from build123d import *

# Parameters (mm, degrees)
F1_DEPTH  = 19.05
F4_DEPTH  = 114.3
F5_W      = 304.8
F5_H      = 76.2
F6_DEPTH  = 205.103861168
F8_DEPTH  = 762
F10_DEPTH = 762
F11_W     = 50.8
F11_H     = 50.8
F12_DEPTH = 762


with BuildPart() as f1:
    # F0 (on Top) → F1 (new body)
    with BuildSketch(Plane.XY):
        Polygon((609.6, 0), (0, 0), (0, -609.6), (76.1936366749, -610.5847488248), (609.6, -76.2), align=None)
    extrude(amount=F1_DEPTH)

    # F3 (on face) → F4 (join)
    with BuildSketch(Plane(origin=(0, 0, 0), x_dir=(1, 0, 0), z_dir=(0, 0, -1))):
        Polygon((584.2, 65.6926060926), (65.7952397089, 585.0482356184), (25.4, 584.5261557366), (25.4, 25.4), (584.2, 25.4), align=None)
        Polygon((44.45, 44.45), (44.45, 565.720772539), (57.9964419843, 565.8958507136), (565.15, 57.8120606621), (565.15, 44.45), align=None, mode=Mode.SUBTRACT)
    extrude(amount=F4_DEPTH)

    # F5 (on face) → F6 (cut)
    with BuildSketch(Plane(origin=(325.4815326726, -324.8856204339, 0), x_dir=(0.7064585835, 0.7077543852, 0), z_dir=(0.7077543852, -0.7064585835, 0))):
        with Locations((0, -57.15)):
            Rectangle(F5_W, F5_H)
    extrude(amount=-F6_DEPTH, mode=Mode.SUBTRACT)

    # F7 (on face) → F8 (join)
    with BuildSketch(Plane(origin=(0, 0, 0), x_dir=(1, 0, 0), z_dir=(0, 0, -1))):
        Polygon((57.9964419843, 565.8958507136), (44.45, 565.8958507136), (44.45, 515.0958507136), (107.8850816302, 515.9157042449), align=None)
    extrude(amount=F8_DEPTH)

    # F9 (on face) → F10 (join)
    with BuildSketch(Plane(origin=(0, 0, 0), x_dir=(1, 0, 0), z_dir=(0, 0, -1))):
        Polygon((565.15, 44.45), (565.15, 57.8120606621), (514.35, 108.7052391219), (514.35, 44.45), align=None)
    extrude(amount=F10_DEPTH)

    # F11 (on face) → F12 (join)
    with BuildSketch(Plane(origin=(0, 0, 0), x_dir=(1, 0, 0), z_dir=(0, 0, -1))):
        with Locations((69.85, 69.85)):
            Rectangle(F11_W, F11_H)
    extrude(amount=F12_DEPTH)


solid = f1.part
Geometry check sheet. Reference: the model listing, model coordinates, mm. A direction names the side the tool comes from. Coordinates: 2 decimals unless noted, no trailing zeros. Order: outer loops, then holes, each group sorted by start corner. A loop starts at its lowest first (then second) coordinate and runs counter-clockwise, first axis right, second up. Notation, with made-up numbers: (75.5, 15.25) - (131.5, 15.25) arc R22 cw to (131.5, 26.25) - close; hole circle Ø6 at (-37, 57.5). An arc over 180 degrees is marked (long way). Answer in a Markdown table with one row per item. Add a question column.
1) Cross-section at A-A, the plane z = -592. Record the cut outline in (x, y).
2) Release check for a two-part mould opening along Y. For faces 6 (the flat face through (534, -70, -762)), 7 (the flat face through (224, -224, 0)), 8 (the flat face through (83.29, -540.556, -433.616)) record: +Y half, -Y half, draft (parallel to the pull), parting line (faces both ways), or undercut.
3) Cross-section at B-B, the plane y = -325.5. Record the cut outline in (x, z), then the cut area to 3 significant figures.
4) Material ranges on line 1 along Z through (x, y) = (81, -341); line 2 along Z through (x, y) = (380.5, -255); line 3 along X through (y, z) = (-211.5, -28.5), recorded low to high. Write a range as [from, to].
5) Set-up check for faces 1 (the flat face through (301, -25.4, -56)), 2 (the flat face through (0, -301, 9)), 3 (the flat face through (540.11, -82.9, -433.62)), 4 (the flat face through (44.45, -69, -434)), 5 (the flat face through (584.2, -45, -56)): record each of +Z, -Z, +X, -X, +Y, -Y from which the full face is reachable in a straight line by a thin tool's end or side.
6) Cross-section at D-D, the plane z = -68. Record the cut outline in (x, y), then the cut area to 3 significant figures.
7) Cross-section at C-C, the plane x = 292.5. Record the cut outline in (y, z).
8) Gauge pin test, flat ends, axial feed: P1, Ø12, axis at x = 486, y = -93.5, coming from the -Z side; P2, Ø11, axis at x = 50, z = -498, coming from the -Y side; P3, Ø14.5, axis at y = -52.5, z = -506.5, coming from the +X side. Record the tip position at first contact, or that the pin passes through.
Check result:
| question | item | result |
|---|---|---|
| 1 | outline | (44.45, -565.9) - (58, -565.9) - (107.89, -515.92) - (44.45, -515.1) - close; (44.45, -95.25) - (95.25, -95.25) - (95.25, -44.45) - (44.45, -44.45) - close; (514.35, -108.71) - (565.15, -57.81) - (565.15, -44.45) - (514.35, -44.45) - close |
| 2 | face 6 | draft |
| 2 | face 7 | undercut |
| 2 | face 8 | -Y half |
| 3 | outline | (0, 0) - (25.4, 0) - (25.4, -114.3) - (44.45, -114.3) - (44.45, 0) - (297.95, 0) - (297.95, -19.05) - (324.87, -19.05) - (324.87, 0) - (360.76, 0) - (360.76, 19.05) - (0, 19.05) - close; (297.95, -114.3) - (324.87, -114.3) - (324.87, -95.25) - (297.95, -95.25) - close |
| 3 | area | 10,100 mm² |
| 4 | line 1 | z = [0, 19.05] |
| 4 | line 2 | z = [-114.3, -95.25], [-19.05, 19.05] |
| 4 | line 3 | x = [25.4, 44.45], [427.61, 438.66] |
| 5 | face 1 | -Z, +X, -X, +Y |
| 5 | face 2 | +Z, -Z, -X, +Y, -Y |
| 5 | face 3 | -Z, +X, -Y |
| 5 | face 4 | -Z, -X, +Y, -Y |
| 5 | face 5 | -Z, +X, +Y, -Y |
| 6 | outline | (25.4, -584.53) - (65.8, -585.05) - (217.82, -432.75) - (204.33, -419.29) - (107.89, -515.92) - (44.45, -515.1) - (44.45, -95.25) - (95.25, -95.25) - (95.25, -44.45) - (514.35, -44.45) - (514.35, -108.71) - (419.66, -203.57) - (433.15, -217.02) - (584.2, -65.69) - (584.2, -25.4) - (25.4, -25.4) - close |
| 6 | area | 36,100 mm² |
| 7 | outline | (-393.88, 0) - (-357.93, 0) - (-357.93, -19.05) - (-330.96, -19.05) - (-330.96, 0) - (-44.45, 0) - (-44.45, -114.3) - (-25.4, -114.3) - (-25.4, 0) - (0, 0) - (0, 19.05) - (-393.88, 19.05) - close; (-357.93, -114.3) - (-330.96, -114.3) - (-330.96, -95.25) - (-357.93, -95.25) - close |
| 8 | P1 | stops at z = 0 |
| 8 | P2 | stops at y = -565.9 |
| 8 | P3 | stops at x = 565.15 |
